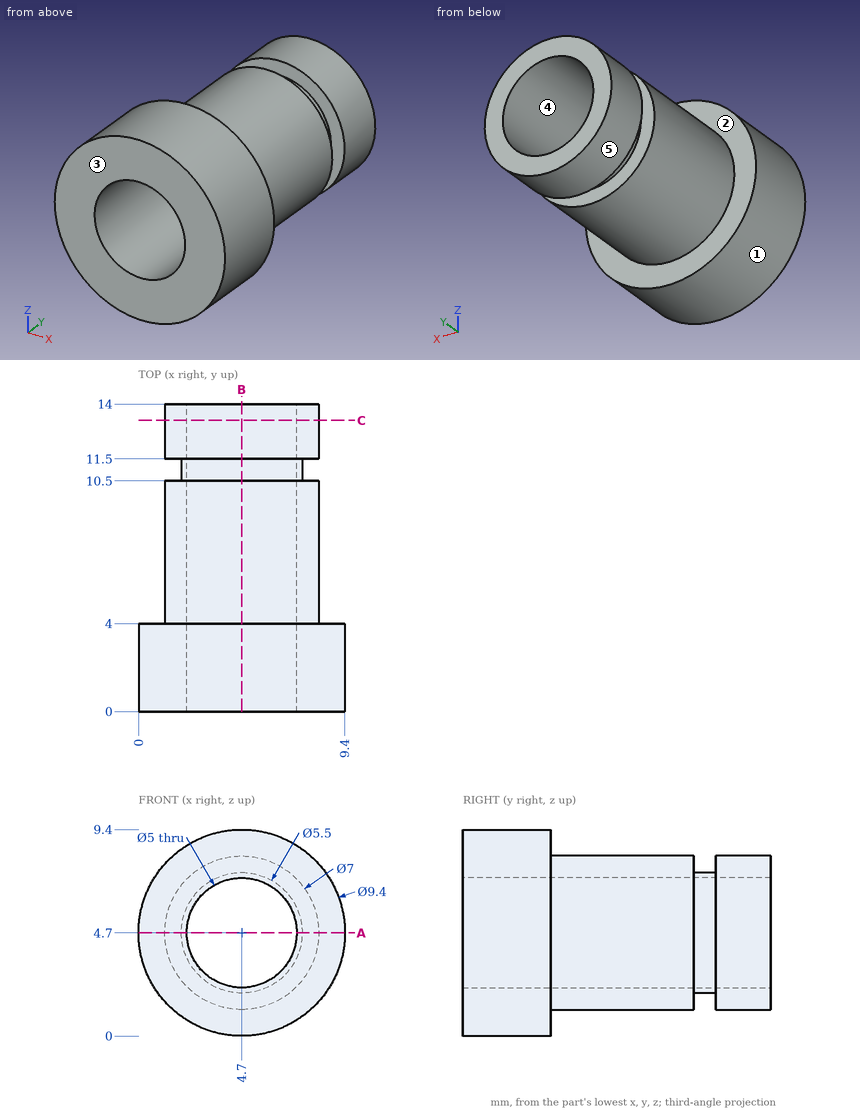
Could you check a few things on this drawing? It's one solid part, dimensions in mm from its lowest x, y, z. A direction names the side the tool comes from. Give positions to 0.01 mm unless a question says otherwise; leave off trailing zeros. Order: outer loops, then holes, each group sorted by start corner. A loop starts at its lowest first (then second) coordinate and runs counter-clockwise, first axis right, second up. Notation, with made-up numbers: (33.25, 2.5) - (45.25, 2.5) arc R27 cw to (45.25, 32.5) - close; hole circle Ø4 at (57.25, -18.75). An arc over 180 degrees is marked (long way). One line per item, written item: value. Start each with the question number.
1. Imagine slicing it at A-A on z = 4.7. List the corners of the cut face in (x, y) for me, plus the area to 3 significant figures.
2. If I drill on probe 1 along Y at (x, z) = (2, 5.5); probe 2 along X at (y, z) = (8.25, 4.7); probe 3 along Y at (x, z) = (6.75, 8.5), over which ranges is the centre line in solid material (lowest first)?
3. For the marked faces 1 and 2, which set-ups out of +Z, -Z, +X, -X, +Y, -Y let a thin tool reach every point of the face, with its end or its side?
4. Imagine slicing it at C-C on y = 13.25. List the corners of the cut face in (x, z) for me.
5. For P1, Ø5, axis at x = 4, y = 9.5, coming from the -Z side; P2, Ø4.5, axis at x = 4.7, z = 4.7, coming from the -Y side, each with a flat end and sliding along its axis, tell me the tip position at first contact or that it passes through.
6. Thinking about a two-plate mould opening in X: for the marked faces 3, 4 and 5, which applies, +X half, -X half, draft (parallel to the pull), parting line (faces both ways), or undercut?
7. Imagine slicing it at B-B on x = 4.7. List the corners of the cut face in (y, z) for me.
Values:
1. outline: (0, 0) - (2.2, 0) - (2.2, 14) - (1.2, 14) - (1.2, 11.5) - (1.95, 11.5) - (1.95, 10.5) - (1.2, 10.5) - (1.2, 4) - (0, 4) - close; (7.2, 0) - (9.4, 0) - (9.4, 4) - (8.2, 4) - (8.2, 10.5) - (7.45, 10.5) - (7.45, 11.5) - (8.2, 11.5) - (8.2, 14) - (7.2, 14) - close
1. area: 36.1 mm²
2. probe 1: 0 to 10.5, 11.5 to 14
2. probe 2: 1.2 to 2.2, 7.2 to 8.2
2. probe 3: 0 to 4
3. face 1: +Y, -Y
3. face 2: +Y
4. outline: circle Ø7 at (4.7, 4.7); hole circle Ø5 at (4.7, 4.7)
5. P1: z = 1.2
5. P2: through
6. face 3: draft
6. face 4: undercut
6. face 5: parting line
7. outline: (0, 0) - (4, 0) - (4, 1.2) - (10.5, 1.2) - (10.5, 1.95) - (11.5, 1.95) - (11.5, 1.2) - (14, 1.2) - (14, 2.2) - (0, 2.2) - close; (0, 7.2) - (14, 7.2) - (14, 8.2) - (11.5, 8.2) - (11.5, 7.45) - (10.5, 7.45) - (10.5, 8.2) - (4, 8.2) - (4, 9.4) - (0, 9.4) - close
